Can you work these out from the model? Positions are in its coordinate system, mm. A direction names the side the tool comes from. Give positions to 0.01 mm unless a question says otherwise; leave off trailing zeros. Loops run counter-clockwise (first coordinate to the right, second up) from the corner with the lowest first, then second, coordinate; pieces in that order, holes last. Notation, with made-up numbers: (69, 60) -> (89, 60) arc R9 cw to (89, 77) -> close; hole circle Ø8 at (66, -7). An arc over 180 degrees is marked (long way). One line per question, with ' | ' between items.
from build123d import *

# Parameters (mm, degrees)
EXTRUDE_1_DEPTH     = 40
SKETCH_2_R          = 3.3
CUT_EXTRUDE_1_DEPTH = 40
SKETCH_3_R          = 3.3
CUT_EXTRUDE_2_DEPTH = 40


with BuildPart() as part:
    # 草图1 → 凸台-拉伸1 (new body)
    with BuildSketch(Plane.XY):
        Polygon((0, 0), (0, 30), (3, 30), (3, 3), (30, 3), (30, 0), align=None)
    extrude(amount=EXTRUDE_1_DEPTH)

    # 草图2 → 切除-拉伸1 (cut)
    with BuildSketch(Plane.ZY):
        with Locations((10, 22)):
            Circle(SKETCH_2_R)
        with Locations((30, 22)):
            Circle(SKETCH_2_R)
    extrude(amount=-CUT_EXTRUDE_1_DEPTH, mode=Mode.SUBTRACT)

    # 草图3 → 切除-拉伸2 (cut)
    with BuildSketch(Plane.XZ):
        with Locations((22, 30)):
            Circle(SKETCH_3_R)
        with Locations((22, 10)):
            Circle(SKETCH_3_R)
    extrude(amount=-CUT_EXTRUDE_2_DEPTH, mode=Mode.SUBTRACT)


solid = part.part
Q1. If we section it at B-B (z = 10): Write out the boundary of the cut face in (x, y), plus the area to 3 significant figures.
Entries:
outline: (0, 0) -> (18.7, 0) -> (18.7, 3) -> (3, 3) -> (3, 18.7) -> (0, 18.7) -> close; (0, 25.3) -> (3, 25.3) -> (3, 30) -> (0, 30) -> close; (25.3, 0) -> (30, 0) -> (30, 3) -> (25.3, 3) -> close | area: 131 mm²
Q2. On a 3-axis mill with a long thin cutter (end or side, diameter ignored), from which of +Z, -Z, +X, -X, +Y, -Y can I reach the whole of each face in a straight line? I mean faces 4 (the face through (3, 17, 20)), 5 (the face through (8.4, 2.8, 40)). Say none if no direction works.
Entries:
face 4: +Z, -Z, +X, +Y | face 5: +Z, +X, -X, +Y, -Y
Q3. If we section it at D-D (z = 15): Write out the boundary of the cut face in (x, y).
Entries:
outline: (0, 0) -> (30, 0) -> (30, 3) -> (3, 3) -> (3, 30) -> (0, 30) -> close
Q4. For pin 1 Ø3 at (y, z) = (10, 7) entering from +X; pin 2 Ø7.5 at (x, z) = (22, 30) entering from +Y, each with a flat end and sliding along its axis, tell me the tip position at first contact or that it passes through.
Entries:
pin 1: x = 3 | pin 2: y = 3
Q5. If we section it at A-A (y = 22): Write out the boundary of the cut face in (x, z), plus the area to 3 significant figures.
Entries:
outline: (0, 0) -> (3, 0) -> (3, 6.7) -> (0, 6.7) -> close; (0, 13.3) -> (3, 13.3) -> (3, 26.7) -> (0, 26.7) -> close; (0, 33.3) -> (3, 33.3) -> (3, 40) -> (0, 40) -> close | area: 80.4 mm²
Q6. If I drill on probe 1 along Z at (x, y) = (22, 1.05); probe 2 along Y at (x, z) = (1.6, 30); probe 3 along Z at (x, y) = (19, 1.5), over which ranges is the centre line in solid material (lowest first)? Write a range as from..to.
Entries:
probe 1: 0..6.7, 13.3..26.7, 33.3..40 | probe 2: 0..18.7, 25.3..30 | probe 3: 0..8.63, 11.37..28.63, 31.37..40
Q7. If we mould it in two halves opening along X, with no side actions, what happens to faces 1 (the face through (15, 0, 20)), 2 (the face through (25.05, 1.48, 28.74)), 3 (the face through (0, 15, 20))? For each: pulls with the +X half, pulls with the -X half, needs draft (parallel to the pull), parting line crosses it, or undercut.
Entries:
face 1: needs draft | face 2: undercut | face 3: pulls with the -X half
